```python
from build123d import *

# Parameters (mm, degrees)
SKETCH1_R           = 23.6982
SKETCH1_R_2         = 22.225
BOSS_EXTRUDE1_DEPTH = 381
CUT_EXTRUDE2_START  = -28.631769
SKETCH3_W           = 3.175
SKETCH3_H           = 89.9999978
CUT_EXTRUDE2_DEPTH  = 1.529969
CIRPATTERN4_COUNT   = 3


with BuildPart() as part:
    # Sketch1 → Boss-Extrude1 (new body)
    with BuildSketch(Plane.XY):
        Circle(SKETCH1_R)
        Circle(SKETCH1_R_2, mode=Mode.SUBTRACT)
    extrude(amount=BOSS_EXTRUDE1_DEPTH)

    # Sketch3 → Cut-Extrude2 (cut)
    with BuildSketch(Plane(origin=(0, 50.8, 0), x_dir=(1, 0, 0), z_dir=(0, 1, 0)).offset(CUT_EXTRUDE2_START)):
        with Locations((0, -315.1720011)):
            Rectangle(SKETCH3_W, SKETCH3_H)
    cut_extrude2 = extrude(amount=CUT_EXTRUDE2_DEPTH, mode=Mode.SUBTRACT)

    # CirPattern4: Cut-Extrude2 ×3 about axis
    cirpattern4_axis = Axis((0, 0, 0), (0, 0, 1))
    for i in range(1, CIRPATTERN4_COUNT):
        add(cut_extrude2.rotate(cirpattern4_axis, i * 360 / CIRPATTERN4_COUNT), mode=Mode.SUBTRACT)


solid = part.part
```
Could you check a few things on this model? Use its own coordinates, in mm. Give positions to 0.01 mm unless a question says otherwise; leave off trailing zeros. Order: outer loops, then holes, each group sorted by start corner. A loop starts at its lowest first (then second) coordinate and runs counter-clockwise, first axis right, second up.
Q1. We'd pull the mould along X, two halves only. Please class faces 1 (the cylindrical face through (-5.137, -23.135, 187.833)), 2 (the cylindrical face through (21.199, 6.676, 187.833)): +X half, -X half, draft (parallel to the pull), parting line (faces both ways), or undercut.
Q2. Suppose I cut it at C-C, the plane x = 11.5. Write out the boundary of the cut face in (y, z).
Q3. If I drill on line 1 along Y through (x, z) = (0, 128) (3 decimals); line 2 along Y through (x, z) = (1.5, 133); line 3 along Y through (x, z) = (0, 274.5) (3 decimals), over which ranges is the centre line in solid material (lowest first)?
Q4. Suppose I cut it at D-D, the plane z = 83. Write out the boundary of the cut face in (x, y) (3 decimals), and give its area (3 significant figures).
Q5. Suppose I cut it at B-B, the plane y = 0. Write out the boundary of the cut face in (x, z) (3 decimals), and give its area (3 significant figures).
Q6. Suppose I cut it at A-A, the plane z = 304.5. Count the separate pieces of the cut face and the enclosed holes in it, and give its area (3 significant figures).
Q7. I'm going to push flat-ended pins straight in: P1, Ø3, axis at x = -2, z = 321, coming from the -Y side; P2, Ø4, axis at x = 16.5, z = 139.5, coming from the -Y side; P3, Ø1, axis at x = 16.5, z = 69.5, coming from the +Y side. Where does each tip first touch, or does it pass through?
Solution:
1. face 1: parting line
1. face 2: undercut
2. outline: (-20.72, 0) - (-19.02, 0) - (-19.02, 381) - (-20.72, 381) - close; (19.02, 0) - (20.72, 0) - (20.72, 381) - (19.02, 381) - close
3. line 1: y = -23.698 to -22.225, 22.225 to 23.698
3. line 2: y = -23.65 to -22.17, 22.17 to 23.65
3. line 3: y = -23.698 to -22.225
4. outline: circle Ø47.396 at (0, 0); hole circle Ø44.45 at (0, 0)
4. area: 213 mm2
5. outline: (-23.698, 0) - (-22.225, 0) - (-22.225, 381) - (-23.698, 381) - close; (22.225, 0) - (23.698, 0) - (23.698, 381) - (22.225, 381) - close
5. area: 1,120 mm2
6. separate pieces: 3
6. enclosed holes: 0
6. area: 198 mm2
7. P1: stops at y = -23.69
7. P2: stops at y = -18.74
7. P3: stops at y = 17.48
